```python
from build123d import *

# Parameters (mm, degrees)
CHAMFER_1_SIZE         = 2
CHAMFER_2_SIZE         = 0.5
HOLE_WIZARD_M61_D      = 6.4
SKETCH_2_R             = 3
CUT_EXTRUDE_1_DEPTH    = 7
SKETCH_4_R             = 21.688
CUT_EXTRUDE_2_DEPTH    = 7.5
PATTERN_LINEAR_1_COUNT = 6
PATTERN_LINEAR_1_PITCH = 1.386


with BuildPart() as part:
    # Эскиз1 → Повернуть1 (revolve)
    with BuildSketch(Plane.XY):
        Polygon((-39.5, 0), (-21, 0), (-21, 20), (-27, 20), (-27, 6), (-39.5, 6), align=None)
    revolve(axis=Axis((0, 0, 0), (0, 1, 0)))

    # Фаска1
    chamfer_1_edges = [part.edges().sort_by_distance(p)[0] for p in [
        (27, 6, 0),
    ]]
    chamfer(chamfer_1_edges, length=CHAMFER_1_SIZE)

    # Фаска2
    chamfer_2_edges = [part.edges().sort_by_distance(p)[0] for p in [
        (39.5, 6, 0),
        (27, 20, 0),
        (39.5, 0, 0),
    ]]
    chamfer(chamfer_2_edges, length=CHAMFER_2_SIZE)

    # Отверстие с зазором M61 (through all)
    with Locations(Plane(origin=(-16.75, 6, 29.011851027), x_dir=(0, 0, 1), z_dir=(0, 1, 0))):
        with Locations((0, 0), (-45.761851027, -12.261851027), (-58.023702054, 33.5), (-12.261851027, 45.761851027), (-12.261851027, -12.261851027), (-58.023702054, 0), (-45.761851027, 45.761851027), (0, 33.5)):
            Hole(HOLE_WIZARD_M61_D / 2)

    # Эскиз2 → Вытянуть1 (cut, through all)
    with BuildSketch(Plane(origin=(0, 6, 0), x_dir=(1, 0, 0), z_dir=(0, 1, 0))):
        with Locations((-33.5, 0)):
            Circle(SKETCH_2_R)
        with Locations((0, 33.5)):
            Circle(SKETCH_2_R)
        with Locations((33.5, 0)):
            Circle(SKETCH_2_R)
        with Locations((0, -33.5)):
            Circle(SKETCH_2_R)
    extrude(amount=-CUT_EXTRUDE_1_DEPTH, mode=Mode.SUBTRACT)

    # Эскиз6 → Вырез-Повернуть2 (revolve, cut)
    with BuildSketch(Plane(origin=(0, 6, 0), x_dir=(1, 0, 0), z_dir=(0, 1, 0))):
        with BuildLine():
            Line((-24.04163056, 24.04163056), (-23.334523779, 23.334523779))
            ThreePointArc((-23.334523779, 23.334523779), (-24.04163056, 23.334523779), (-24.04163056, 24.04163056))
        make_face()
    revolve(axis=Axis((0, 6, 0), (-0.707106781, 0, -0.707106781)), mode=Mode.SUBTRACT)

    # Эскиз4 → Вытянуть2 (cut)
    with BuildSketch(Plane(origin=(0, 20, 0), x_dir=(1, 0, 0), z_dir=(0, 1, 0))):
        Circle(SKETCH_4_R)
    extrude(amount=-CUT_EXTRUDE_2_DEPTH, mode=Mode.SUBTRACT)

    # Эскиз5 → Вырез-Повернуть1 (revolve, cut)
    with BuildSketch(Plane.XY):
        Polygon((-22.5, 20), (-21.688, 20.568568521), (-15, 20.568568521), (-15, 19.431431479), (-21.688, 19.431431479), align=None)
    cut_revolve_1 = revolve(axis=Axis((0, 0, 0), (0, 1, 0)), mode=Mode.SUBTRACT)

    # Линейный массив1: Вырез-Повернуть1 ×6
    with Locations(*[(0, -i * PATTERN_LINEAR_1_PITCH, 0) for i in range(1, PATTERN_LINEAR_1_COUNT)]):
        add(cut_revolve_1, mode=Mode.SUBTRACT)


solid = part.part
```
Verification items for the finished model (mm, model axes). Coordinates: 2 decimals unless noted, no trailing zeros. Write each loop counter-clockwise with the first axis right and the second up, starting at its lowest first coordinate (ties: lowest second). Pieces come first, ordered by that corner, then holes. Notation, with made-up numbers: (-16.75, -38.75) - (29.25, -38.75) arc R13 ccw to (29.25, -17.75) - close; hole circle Ø8 at (50, 82). An arc over 180 degrees is marked (long way). Write item = value, one per line.
Q1. Cross-section at C-C (y = 11.25). Enter the section's corners in (x, z).
Answer:
outline = circle Ø54 at (0, 0); hole circle Ø42 at (0, 0)
Q2. Cross-section at A-A (x = 0). Give the number of separate pieces and of enclosed holes in the cut face, plus the area to 3 significant figures.
Answer:
separate_pieces = 4
enclosed_holes = 0
area = 306 mm²
Q3. Go/stop test with flat-tipped pins: pin 1 Ø8 at (y, z) = (4.5, 27) entering from -X; pin 2 Ø10 at (x, z) = (-27, 2) entering from -Y; pin 3 Ø5 at (x, y) = (8.5, 15) entering from -Z; pin 4 Ø3.5 at (x, z) = (33.5, 0) entering from +Y. Record where each tip stops, or that it passes through.
Answer:
pin_1 = -32.11
pin_2 = 0
pin_3 = -26.32
pin_4 = through
Q4. Material ranges on L1, parallel to Z at x = 0, y = 5; L2, parallel to Z at x = -19, y = 4.75; L3, parallel to Z at x = 0, y = 19.35, recorded low to high. Write a range as from..to.
Answer:
L1 = -39.5..-36.5, -30.5..-21, 21..30.5, 36.5..39.5
L2 = -34.63..-31.29, -26.74..-8.94, 8.94..26.74, 31.29..34.63
L3 = -27..-21.69, 21.69..27
